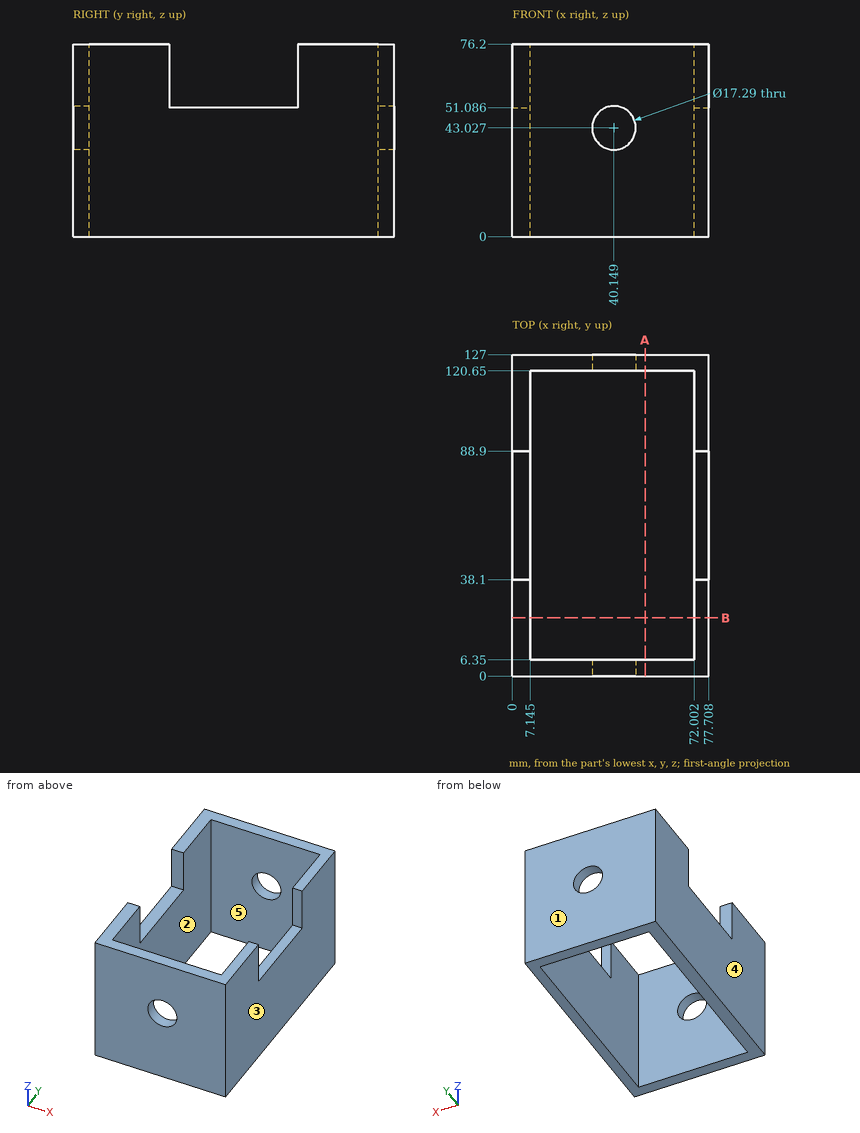
Design review of the part shown in the three views and the two pictorial views. Dimensions are in mm from the part's minimum x, y and z. A direction names the side the tool comes from. Round coordinates to 2 decimals unless told otherwise and drop trailing zeros. Loops run counter-clockwise (first coordinate to the right, second up) from the corner with the lowest first, then second, coordinate; pieces in that order, holes last. Notation, with made-up numbers: (74, -11.75) - (86, -11.75) arc R16 ccw to (86, 14.25) - close; hole circle Ø10 at (81, 35.5). An arc over 180 degrees is marked (long way). Answer as CSV lines item,"result".
(1) Consider section A-A on x = 52.5. Give the boundary of the cut face in (y, z).
Checked values:
outline,"(0, 0) - (6.35, 0) - (6.35, 76.2) - (0, 76.2) - close; (120.65, 0) - (127, 0) - (127, 76.2) - (120.65, 76.2) - close"
(2) Tool access review of the marked faces 1 and 2: name each direction out of +Z, -Z, +X, -X, +Y, -Y from which nothing blocks a thin tool from reaching the whole face with its end or side.
Checked values:
face 1,"+Z, -Z, +X, -X, +Y"
face 2,"+Z, -Z"
(3) Wall thickness on line 1 (X direction, y = 7, z = 26) (1 decimal); line 2 (Y direction, x = 48.5, z = 57); line 3 (Z direction, x = 6, y = 66) (1 decimal): over which ranges is each line inside the solid? List them lowest first.
Checked values:
line 1,"x = 0 to 7.1, 72 to 77.7"
line 2,"y = 0 to 6.35, 120.65 to 127"
line 3,"z = 0 to 51.1"
(4) Consider section B-B on y = 23. Give the boundary of the cut face in (x, z) (1 decimal).
Checked values:
outline,"(0, 0) - (7.1, 0) - (7.1, 76.2) - (0, 76.2) - close; (72, 0) - (77.7, 0) - (77.7, 76.2) - (72, 76.2) - close"
(5) Insertion check: P1, Ø8, axis at x = 3, y = 62, coming from the +Z side. The pin has a flat end and moves straight along its axis. Give the tip position at first contact, or say it passes through.
Checked values:
P1,"stops at z = 51.09"
(6) Mouldability with a two-part tool opening along X and no side actions: class the marked faces 3, 4 and 5 as +X half, -X half, draft (parallel to the pull), parting line (faces both ways), or undercut.
Checked values:
face 3,"+X half"
face 4,"-X half"
face 5,"undercut"
